```python
from build123d import *

# Parameters (mm, degrees)
F1_DEPTH = 5.6
F3_DEPTH = 2.5
F5_DEPTH = 2.5


with BuildPart() as f1:
    # F0 (on Top) → F1 (new body)
    with BuildSketch(Plane.XY):
        Polygon((25, 3.75), (0, 3.75), (-25, 3.75), (-25, 2.05), (-27.5, 2.05), (-27.5, 3.05), (-29.5, 1.1), (-25, 1.1), (-25, -1.1), (-29.5, -1.1), (-27.5, -3.05), (-27.5, -2.05), (-25, -2.05), (-25, -3.75), (0, -3.75), (25, -3.75), (25, -2.05), (27.5, -2.05), (27.5, -3.05), (29.5, -1.1), (25, -1.1), (25, 1.1), (29.5, 1.1), (27.5, 3.05), (27.5, 2.05), (25, 2.05), align=None)
    extrude(amount=F1_DEPTH)

    # F2 (on face) → F3 (cut)
    with BuildSketch(Plane.XY.offset(5.6)):
        Polygon((22.5, -1.25), (22.5, 1), (22.5, 1.25), (-22.5, 1.25), (-22.5, -1), (-22.5, -1.25), align=None)
    extrude(amount=-F3_DEPTH, mode=Mode.SUBTRACT)

    # F4 (on face) → F5 (cut)
    with BuildSketch(Plane(origin=(0, 0, 0), x_dir=(1, 0, 0), z_dir=(0, 0, -1))):
        Polygon((-22.5, 1.25), (-22.5, 0.4), (-22.5, -1.25), (22.5, -1.25), (22.5, -0.4), (22.5, 1.25), align=None)
    extrude(amount=-F5_DEPTH, mode=Mode.SUBTRACT)


solid = f1.part
```
Geometry check sheet. Reference: the model listing, model coordinates, mm. A direction names the side the tool comes from. Give positions to 0.01 mm unless a question says otherwise; leave off trailing zeros. Loops run counter-clockwise (first coordinate to the right, second up) from the corner with the lowest first, then second, coordinate; pieces in that order, holes last. Notation, with made-up numbers: M 44,23 L 55,23 A29 cw 55,44 Z; hole C 70,28.25 d1. An arc over 180 degrees is marked long. Write item = value, one per line. Start each with the question number.
1. Section check A-A, the plane z = 1.55. Enter the section's corners in (x, y).
2. Go/stop test with flat-tipped pins: P1, Ø0.5, axis at y = 2.5, z = 2.5, coming from the -X side; P2, Ø0.5, axis at y = -3, z = 3, coming from the +X side; P3, Ø1.3, axis at x = -27.5, z = 3.5, coming from the +Y side. Record where each tip stops, or that it passes through.
3. Section check B-B, the plane y = -0.5. Enter the section's corners in (x, z).
4. Tool access check on faces 1 (the face through (-26, 2.05, 3)), 2 (the face through (22.5, 0, 4)), 3 (the face through (26, -2.05, 3)), 4 (the face through (0, 1.25, 1)). Record the directions out of +Z, -Z, +X, -X, +Y, -Y that give a thin tool (end or side, any length) a straight path to the whole face; none if there is none.
5. Thickness scan on probe 1 along Y at (x, z) = (12, 3.7); probe 2 along X at (y, z) = (-1, 1.05); probe 3 along X at (y, z) = (2.25, 1.1). Record the ranges inside material, lowest first.
6. Draft check along Y on faces 5 (the face through (26, 2.05, 3)), 6 (the face through (25, -3, 3)), 7 (the face through (-22.5, 0, 4)). Enter one of: +Y half, -Y half, draft (parallel to the pull), parting line (faces both ways), or undercut.
7. Section check C-C, the plane x = 12.5. Enter the section's corners in (y, z), plus the area to 3 significant figures.
Values follow:
q1.outline = M -29.5,-1.1 L -27.5,-3.05 L -27.5,-2.05 L -25,-2.05 L -25,-3.75 L 25,-3.75 L 25,-2.05 L 27.5,-2.05 L 27.5,-3.05 L 29.5,-1.1 L 25,-1.1 L 25,1.1 L 29.5,1.1 L 27.5,3.05 L 27.5,2.05 L 25,2.05 L 25,3.75 L -25,3.75 L -25,2.05 L -27.5,2.05 L -27.5,3.05 L -29.5,1.1 L -25,1.1 L -25,-1.1 Z; hole M -22.5,-1.25 L 22.5,-1.25 L 22.5,1.25 L -22.5,1.25 Z
q2.P1 = -28.32
q2.P2 = 27.81
q2.P3 = 3.05
q3.outline = M -25,0 L -22.5,0 L -22.5,2.5 L 22.5,2.5 L 22.5,0 L 25,0 L 25,5.6 L 22.5,5.6 L 22.5,3.1 L -22.5,3.1 L -22.5,5.6 L -25,5.6 Z
q4.face_1 = +Z, -Z, +Y
q4.face_2 = +Z
q4.face_3 = +Z, -Z, -Y
q4.face_4 = -Z
q5.probe_1 = -3.75 to -1.25, 1.25 to 3.75
q5.probe_2 = -25 to -22.5, 22.5 to 25
q5.probe_3 = -28.32 to -27.5, -25 to 25, 27.5 to 28.32
q6.face_5 = +Y half
q6.face_6 = draft
q6.face_7 = undercut
q7.outline = M -3.75,0 L -1.25,0 L -1.25,2.5 L 1.25,2.5 L 1.25,0 L 3.75,0 L 3.75,5.6 L 1.25,5.6 L 1.25,3.1 L -1.25,3.1 L -1.25,5.6 L -3.75,5.6 Z
q7.area = 29.5 mm^2
